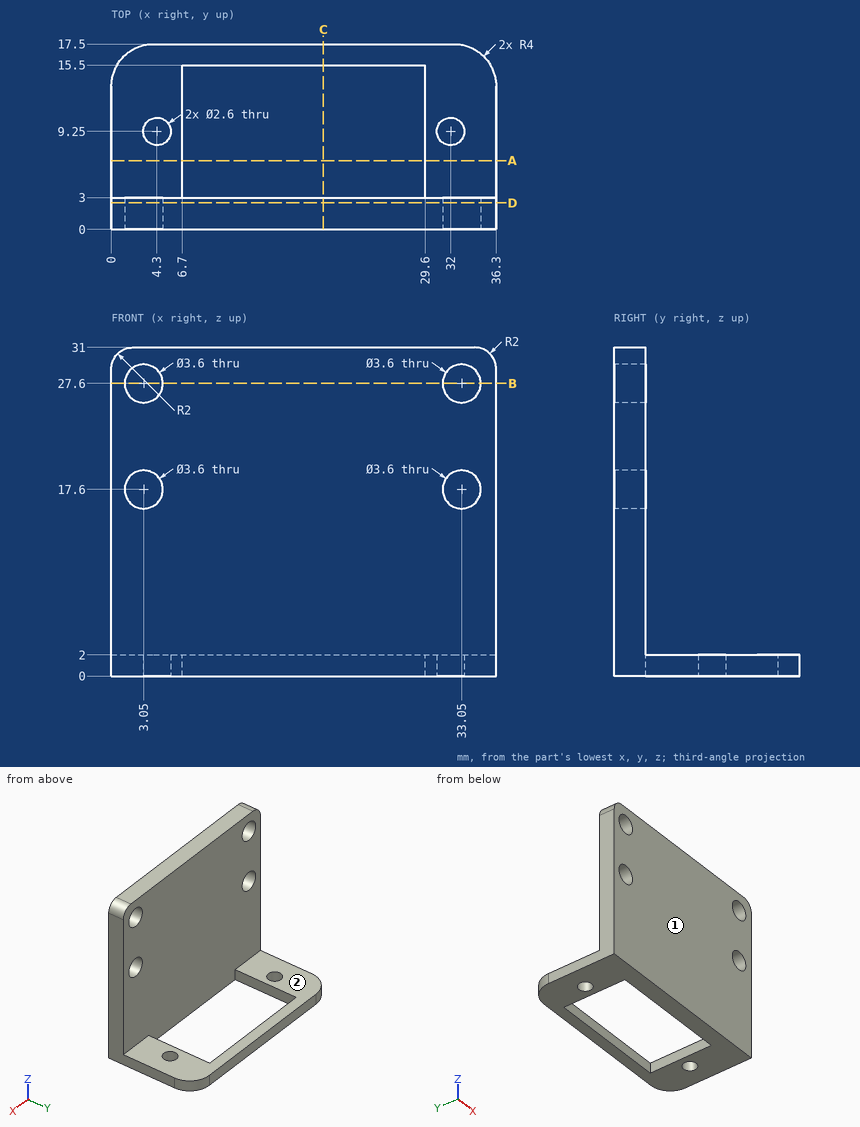
Input: dimensioned drawing with shaded views. Units: mm. Origin: part minimum x, y, z. A direction names the side the tool comes from. Coordinates: 2 decimals unless noted, no trailing zeros. Order: outer loops, then holes, each group sorted by start corner. A loop starts at its lowest first (then second) coordinate and runs counter-clockwise, first axis right, second up.
(1) Material intervals for probe 1 along X at (y, z) = (1.5, 17.6); probe 2 along Y at (x, z) = (32, 1); probe 3 along Z at (x, y) = (2.5, 16), sorted ascending.
(2) Access query for the marked faces 1 and 2. Directions: +Z, -Z, +X, -X, +Y, -Y. A direction counts if a zero-diameter tool reaches every point of the face in a straight line with its end or side. Return the directions, or none.
(3) Section query D-D (y = 2.5). Return the cut outline in (x, z), plus the area to 3 significant figures.
(4) Section query B-B (z = 27.6). Return the cut outline in (x, y).
(5) First-contact query: pin 1 (5 mm diameter, centred on x = 7.5, y = 4, fed in from +Z); pin 2 (3 mm diameter, centred on x = 23, z = 24.5, fed in from +Y). Flat tips, straight axial feed; report the tip coordinate or a pass-through.
(6) Section query A-A (y = 6.5). Return the cut outline in (x, z), plus the area to 3 significant figures.
(7) Section query C-C (x = 20). Return the cut outline in (y, z).
Solution:
1. probe 1: x = 0 to 1.25, 4.85 to 31.25, 34.85 to 36.3
1. probe 2: y = 0 to 7.95, 10.55 to 17.5
1. probe 3: z = 0 to 2
2. face 1: +Z, -Z, +X, -X, -Y
2. face 2: +Z, +X, -X, +Y
3. outline: (0, 0) - (36.3, 0) - (36.3, 29) arc R2 ccw to (34.3, 31) - (2, 31) arc R2 ccw to (0, 29) - close; hole circle Ø3.6 at (3.05, 17.6); hole circle Ø3.6 at (3.05, 27.6); hole circle Ø3.6 at (33.05, 17.6); hole circle Ø3.6 at (33.05, 27.6)
3. area: 1,080 mm2
4. outline: (0, 0) - (1.25, 0) - (1.25, 3) - (0, 3) - close; (4.85, 0) - (31.25, 0) - (31.25, 3) - (4.85, 3) - close; (34.85, 0) - (36.3, 0) - (36.3, 3) - (34.85, 3) - close
5. pin 1: stops at z = 31
5. pin 2: stops at y = 3
6. outline: (0, 0) - (6.7, 0) - (6.7, 2) - (0, 2) - close; (29.6, 0) - (36.3, 0) - (36.3, 2) - (29.6, 2) - close
6. area: 26.8 mm2
7. outline: (0, 0) - (3, 0) - (3, 31) - (0, 31) - close; (15.5, 0) - (17.5, 0) - (17.5, 2) - (15.5, 2) - close
